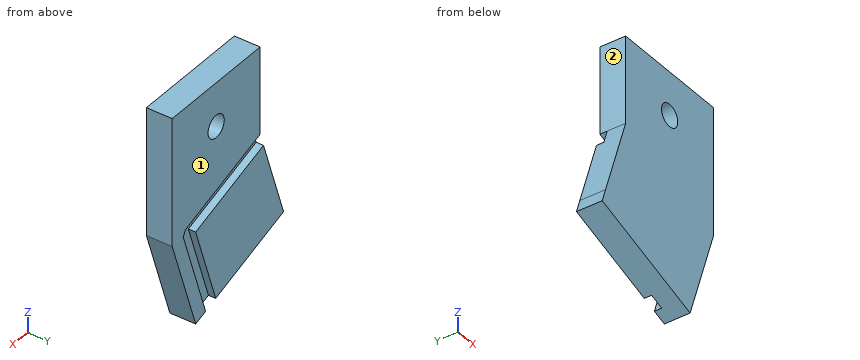
Autodesk Inventor part; units mm, degrees
ref_plane "YZ Plane" through (0, 0, 0) normal (1, 0, 0) x (0, 1, 0)
ref_plane "XZ Plane" through (0, 0, 0) normal (0, 1, 0) x (-1, 0, 0)
ref_plane "XY Plane" through (0, 0, 0) normal (0, 0, 1) x (1, 0, 0)
sketch "Sketch1" plane through (0, 0, 0) normal (0, 1, 0) x (-1, 0, 0)
  line L0 (-8.0312, -19.6194) -> (-8.0312, -0.5694)
  line L1 (-8.0312, -0.5694) -> (-34.5277, -0.5694)
  line L2 (-34.5277, -0.5694) -> (-34.5277, -28.5056)
  line L3 (18.6455, 5.0782) -> (18.6456, 5.0782)
  line L4 (-1.974, -37.6808) -> (-8.0312, -19.6194)
  line L5 (-34.5277, -28.5056) -> (-27.4611, -49.5771)
  line L6 (-1.974, -37.6808) -> (-0.9645, -40.691)
  line L7 (-27.4611, -49.5771) -> (-0.9645, -40.691)
  circle A0 centre (-21.2794, -10.0945) radius 2.4447
  line L8 (-8.0312, -0.5694) -> (-8.0312, -19.6194)
  line L9 (-8.0312, -19.6194) -> (-0.9645, -40.691)
  line L10 (-0.9645, -40.691) -> (-27.4611, -49.5771)
  line L11 (-27.4611, -49.5771) -> (-34.5277, -28.5056)
  line L12 (-34.5277, -28.5056) -> (-34.5277, -0.5694)
  line L13 (-34.5277, -0.5694) -> (-8.0312, -0.5694)
  point P0 (0, 0)
  dimension "d0" = 19.05
  dimension "d1" = 22.225
  dimension "d2" = 27.9469
  dimension "d3" = 26.4965
  dimension "d4" = 4.8895
extrude "Extrusion1" add sketch "Sketch1" along normal blind 5.6134
sketch "Sketch2" plane through (0, 5.6134, 0) normal (0, 1, 0) x (1, 0, 0)
  line L0 (31.5176, 27.4961) -> (8.0312, 19.6194)
  line L1 (8.0312, 19.6194) -> (7.0136, 22.6537)
  line L2 (7.0136, 22.6537) -> (27.4657, 29.5128)
  line L3 (31.5176, 27.4961) -> (29.9884, 26.9832)
  line L4 (27.4657, 29.5128) -> (21.4165, 47.5499)
  line L5 (21.4165, 47.5499) -> (24.4508, 48.5676)
  line L6 (24.4508, 48.5676) -> (31.5176, 27.4961)
  line L7 (27.4611, 49.5771) -> (0.9645, 40.691)
  point P0 (0, 0)
  point P1 (0, 0)
  dimension "d10" = 3.175
  dimension "d11" = 3.2004
  dimension "d12" = 3.2004
  dimension "d15" = 0
extrude "Extrusion2" cut sketch "Sketch2" against normal blind 1.5875
fillet "Fillet1" radius 1.5875 1 edges at (31.5176, 4.8197, -27.4961)
properties part number "Lidar Sensor Case Piece 2"
Geometry check sheet. Reference: the model listing, model coordinates, mm. Face numbers are marked on the shaded views. A direction names the side the tool comes from. Give positions to 0.01 mm unless a question says otherwise; leave off trailing zeros. Order: outer loops, then holes, each group sorted by start corner. A loop starts at its lowest first (then second) coordinate and runs counter-clockwise, first axis right, second up.
1. Section check C-C, the plane x = 17. Enter the section's corners in (y, z).
2. Section check A-A, the plane y = 4.65. Enter the section's corners in (x, z) (1 decimal).
3. Gauge pin test, flat ends, axial feed: pin 1 Ø3 at (x, z) = (21.28, -10.09) entering from +Y; pin 2 Ø1.5 at (x, y) = (7.5, 2) entering from -Z; pin 3 Ø1 at (x, y) = (5, 4) entering from -Z. Record the tip position at first contact, or that the pin passes through.
4. Access from +Z, -Z, +X, -X, +Y, -Y to the whole of each face (thin tool, end or side, straight path). Record for the marked faces 1 and 2.
5. Section check B-B, the plane z = -12. Enter the section's corners in (x, y).
6. Section check D-D, the plane z = -3.5. Enter the section's corners in (x, y).
7. Thickness scan on L1, parallel to X at y = 2.95, z = -10; L2, parallel to Y at x = 16.5, z = -24.5; L3, parallel to X at y = 1.05, z = -19. Record the ranges inside material, lowest first.
Values follow:
1. outline: (0, -46.07) - (5.61, -46.07) - (5.61, -26) - (4.03, -26) - (4.03, -22.63) - (5.61, -22.63) - (5.61, -0.57) - (0, -0.57) - close
2. outline: (1, -40.7) - (21.4, -47.5) - (27.5, -29.5) - (7, -22.7) - (2, -37.7) - close; (8, -19.6) - (30, -27) arc R1.6 cw to (31, -29) - (24.5, -48.6) - (27.5, -49.6) - (34.5, -28.5) - (34.5, -0.6) - (8, -0.6) - close; hole circle Ø4.9 at (21.3, -10.1)
3. pin 1: passes through
3. pin 2: stops at z = -43.13
3. pin 3: stops at z = -42.21
4. face 1: +Z, -Z, +X, -X, +Y
4. face 2: +Z, -X, +Y, -Y
5. outline: (8.03, 0) - (19.75, 0) - (19.75, 5.61) - (8.03, 5.61) - close; (22.81, 0) - (34.53, 0) - (34.53, 5.61) - (22.81, 5.61) - close
6. outline: (8.03, 0) - (34.53, 0) - (34.53, 5.61) - (8.03, 5.61) - close
7. L1: x = 8.03 to 18.84, 23.72 to 34.53
7. L2: y = 0 to 4.03
7. L3: x = 8.03 to 34.53
